Geometry: final body of the model. Coordinates: model frame, mm. Coordinates: 2 decimals unless noted, no trailing zeros. Write each loop counter-clockwise with the first axis right and the second up, starting at its lowest first coordinate (ties: lowest second). Pieces come first, ordered by that corner, then holes. Notation, with made-up numbers: (39, -20) -> (63, -20) arc R20 ccw to (63, 10) -> close; hole circle Ø5 at (-28, -35). An arc over 180 degrees is marked (long way). One line per item, written item: value.
```python
from build123d import *

# Parameters (mm, degrees)
SKETCH_W   = 117
SKETCH_H   = 42.5
SKETCH_R   = 11.25
SKETCH_R_2 = 4
SKETCH_R_3 = 1.5
PAD_DEPTH  = 3


with BuildPart() as part:
    # Sketch → Pad (new body)
    with BuildSketch(Plane.XY):
        Rectangle(SKETCH_W, SKETCH_H)
        with Locations((-29.25, 0)):
            Circle(SKETCH_R, mode=Mode.SUBTRACT)
        with Locations((29.25, 0)):
            Circle(SKETCH_R, mode=Mode.SUBTRACT)
        Circle(SKETCH_R_2, mode=Mode.SUBTRACT)
        with Locations((-45, 15.5)):
            Circle(SKETCH_R_3, mode=Mode.SUBTRACT)
        with Locations((-14, 15.5)):
            Circle(SKETCH_R_3, mode=Mode.SUBTRACT)
        with Locations((-14, -15.5)):
            Circle(SKETCH_R_3, mode=Mode.SUBTRACT)
        with Locations((-45, -15.5)):
            Circle(SKETCH_R_3, mode=Mode.SUBTRACT)
        with Locations((14, 15.5)):
            Circle(SKETCH_R_3, mode=Mode.SUBTRACT)
        with Locations((45, 15.5)):
            Circle(SKETCH_R_3, mode=Mode.SUBTRACT)
        with Locations((45, -15.5)):
            Circle(SKETCH_R_3, mode=Mode.SUBTRACT)
        with Locations((14, -15.5)):
            Circle(SKETCH_R_3, mode=Mode.SUBTRACT)
    extrude(amount=PAD_DEPTH)


solid = part.part
```
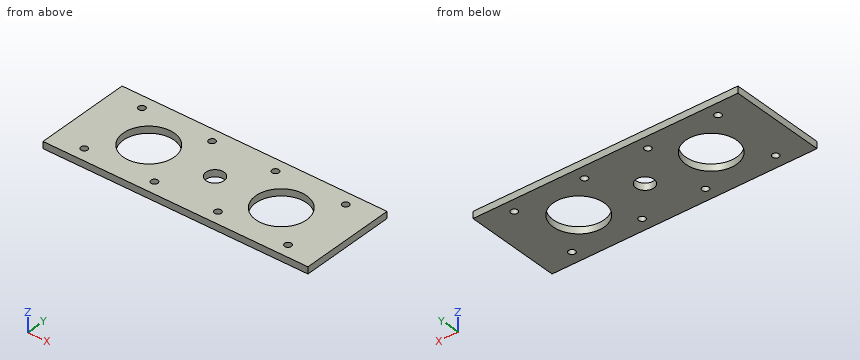
(1) Line query: line 1 (Y direction, x = 14, z = 1.55); line 2 (X direction, y = -15, z = 1.7); line 3 (X direction, y = -5, z = 2). Output: solid intervals per line, ascending. Write a range as [from, to].
Responses:
line 1: y = [-21.25, -17], [-14, 14], [17, 21.25]
line 2: x = [-58.5, -46.41], [-43.59, -15.41], [-12.59, 12.59], [15.41, 43.59], [46.41, 58.5]
line 3: x = [-58.5, -39.33], [-19.17, 19.17], [39.33, 58.5]
(2) Section C-C (z = 1.4). State how many separate pieces and enclosed holes the cut face has, then the cut area to 3 significant figures.
Responses:
separate pieces: 1
enclosed holes: 11
area: 4,070 mm2
(3) Section D-D (y = -15.5). Return the cut outline in (x, z).
Responses:
outline: (-58.5, 0) -> (-46.5, 0) -> (-46.5, 3) -> (-58.5, 3) -> close; (-43.5, 0) -> (-15.5, 0) -> (-15.5, 3) -> (-43.5, 3) -> close; (-12.5, 0) -> (12.5, 0) -> (12.5, 3) -> (-12.5, 3) -> close; (15.5, 0) -> (43.5, 0) -> (43.5, 3) -> (15.5, 3) -> close; (46.5, 0) -> (58.5, 0) -> (58.5, 3) -> (46.5, 3) -> close
(4) Section B-B (x = -45). Return the cut outline in (y, z), then the cut area to 4 significant figures.
Responses:
outline: (-21.25, 0) -> (-17, 0) -> (-17, 3) -> (-21.25, 3) -> close; (-14, 0) -> (14, 0) -> (14, 3) -> (-14, 3) -> close; (17, 0) -> (21.25, 0) -> (21.25, 3) -> (17, 3) -> close
area: 109.5 mm2
(5) Section A-A (x = 29.25). Return the cut outline in (y, z), then the cut area to 3 significant figures.
Responses:
outline: (-21.25, 0) -> (-11.25, 0) -> (-11.25, 3) -> (-21.25, 3) -> close; (11.25, 0) -> (21.25, 0) -> (21.25, 3) -> (11.25, 3) -> close
area: 60.0 mm2
(6) First-contact query: pin 1 (3.5 mm diameter, centred on x = 14, y = 15.5, fed in from +Z). Flat tip, straight axial feed; report the tip coordinate or a pass-through.
Responses:
pin 1: stops at z = 3
